Can you work these out from the model? Positions are in its coordinate system, mm. A direction names the side the tool comes from. Round coordinates to 2 decimals unless told otherwise and drop trailing zeros. Loops run counter-clockwise (first coordinate to the right, second up) from the corner with the lowest first, then second, coordinate; pieces in that order, holes last. Notation, with made-up numbers: (13.5, -11.75) -> (23.5, -11.75) arc R14 ccw to (23.5, -3.75) -> close; hole circle Ø1 at (24, 38). An arc over 180 degrees is marked (long way). Answer as a JSON object with one key per item and string values.
```python
from build123d import *

# Parameters (mm, degrees)
BOSS_EXTRUDE1_DEPTH = 80
SKETCH4_R           = 17.653500843
BOSS_EXTRUDE2_DEPTH = 10
SKETCH5_R           = 5.034978738
BOSS_EXTRUDE3_DEPTH = 17
SKETCH9_R           = 7
BOSS_EXTRUDE6_DEPTH = 0.5


with BuildPart() as part:
    # Sketch3 → Boss-Extrude1 (new body)
    with BuildSketch(Plane.XY):
        with BuildLine():
            Line((-3.371320853, -9.414573581), (-3.371320853, -17.114573581))
            Line((-3.371320853, -17.114573581), (4.328679147, -17.114573581))
            Line((4.328679147, -17.114573581), (4.328679147, -9.014573581))
            ThreePointArc((4.328679147, -9.014573581), (10, 0), (4.328679147, 9.014573581))
            Line((4.328679147, 9.014573581), (4.328679147, 17.114573581))
            Line((4.328679147, 17.114573581), (-3.371320853, 17.114573581))
            Line((-3.371320853, 17.114573581), (-3.371320853, 9.414573581))
            ThreePointArc((-3.371320853, 9.414573581), (-10, 0), (-3.371320853, -9.414573581))
        make_face()
    extrude(amount=BOSS_EXTRUDE1_DEPTH)

    # Sketch4 → Boss-Extrude2 (add)
    with BuildSketch(Plane.XY.offset(80)):
        with Locations(Location((0, 0, 0), (0, 0, 284.1937898))):
            Circle(SKETCH4_R)
    extrude(amount=BOSS_EXTRUDE2_DEPTH)

    # Sketch5 → Boss-Extrude3 (add)
    with BuildSketch(Plane(origin=(0, 0, 0), x_dir=(-1, 0, 0), z_dir=(0, 0, -1))):
        with Locations(Location((0, 0, 0), (0, 0, 180))):
            Circle(SKETCH5_R)
    extrude(amount=BOSS_EXTRUDE3_DEPTH)

    # Sketch9 → Boss-Extrude6 (add)
    with BuildSketch(Plane(origin=(0, 0, -17), x_dir=(-1, 0, 0), z_dir=(0, 0, -1))):
        Circle(SKETCH9_R)
    extrude(amount=BOSS_EXTRUDE6_DEPTH)


solid = part.part
```
Q1. I'm going to push flat-ended pins straight in: pin 1 (4 mm diameter, centred on y = 8, z = 19, fed in from -X); pin 2 (6.5 mm diameter, centred on y = -11.5, z = 22.5, fed in from +X); pin 3 (6 mm diameter, centred on x = 11, y = -12.5, fed in from -Z); pin 4 (17.5 mm diameter, centred on x = -10, y = -2.5, fed in from -Z). Where does each tip first touch, or does it pass through?
Determined:
{"pin 1": "x = -8", "pin 2": "x = 5.65", "pin 3": "z = 80", "pin 4": "z = -17.5"}
Q2. We'd pull the mould along Z, two halves only. Please class faces 5 (the flat face through (12, -2, 80)), 6 (the flat face through (2, 5, -17)), 7 (the flat face through (4, -4, 0)), 8 (the flat face through (0, -17.115, 39)): pulls with the +Z half, pulls with the -Z half, needs draft (parallel to the pull), parting line crosses it, or undercut.
Determined:
{"face 5": "pulls with the -Z half", "face 6": "undercut", "face 7": "undercut", "face 8": "needs draft"}
Q3. I want a section at B-B, the plane z = 46.5. Write out the boundary of the cut face in (x, y), then the cut area to 3 significant figures.
Determined:
{"outline": "(-3.37, -17.11) -> (4.33, -17.11) -> (4.33, -9.01) arc R10 ccw to (4.33, 9.01) -> (4.33, 17.11) -> (-3.37, 17.11) -> (-3.37, 9.41) arc R10 ccw to (-3.37, -9.41) -> close", "area": "428 mm²"}
Q4. I want a section at A-A, the plane x = 6. Write out the boundary of the cut face in (y, z).
Determined:
{"outline": "(-16.6, 80) -> (-8, 80) -> (-8, 0) -> (8, 0) -> (8, 80) -> (16.6, 80) -> (16.6, 90) -> (-16.6, 90) -> close; (-3.61, -17.5) -> (3.61, -17.5) -> (3.61, -17) -> (-3.61, -17) -> close"}
Q5. On a 3-axis mill with a long thin cutter (end or side, diameter ignored), from which of +Z, -Z, +X, -X, +Y, -Y can I reach the whole of each face in a straight line? I mean faces 1 (the flat face through (-3.371, -13, 39)), 2 (the cylindrical face through (-10, 0, 39)), 3 (the flat face through (1, 17.115, 39)), 4 (the flat face through (4.329, -13, 39)). Say none if no direction works.
Determined:
{"face 1": "-Z, -X, -Y", "face 2": "-Z, -X", "face 3": "-Z, +X, -X, +Y", "face 4": "-Z, +X, -Y"}
Q6. I want a section at D-D, the plane y = -13.5. Write out the boundary of the cut face in (x, z).
Determined:
{"outline": "(-11.38, 80) -> (-3.37, 80) -> (-3.37, 0) -> (4.33, 0) -> (4.33, 80) -> (11.38, 80) -> (11.38, 90) -> (-11.38, 90) -> close"}
Q7. I want a section at C-C, the plane x = 0. Write out the boundary of the cut face in (y, z).
Determined:
{"outline": "(-17.65, 80) -> (-17.11, 80) -> (-17.11, 0) -> (-5.03, 0) -> (-5.03, -17) -> (-7, -17) -> (-7, -17.5) -> (7, -17.5) -> (7, -17) -> (5.03, -17) -> (5.03, 0) -> (17.11, 0) -> (17.11, 80) -> (17.65, 80) -> (17.65, 90) -> (-17.65, 90) -> close"}
Q8. If I drill on L1, parallel to Z at x = 1, y = 6.5; L2, parallel to X at y = 13, z = 38; L3, parallel to Z at x = 6.5, y = -5, over which ranges is the centre line in solid material (lowest first)? Write a range as [from, to].
Determined:
{"L1": "[-17.5, -17], [0, 90]", "L2": "[-3.37, 4.33]", "L3": "[0, 90]"}
